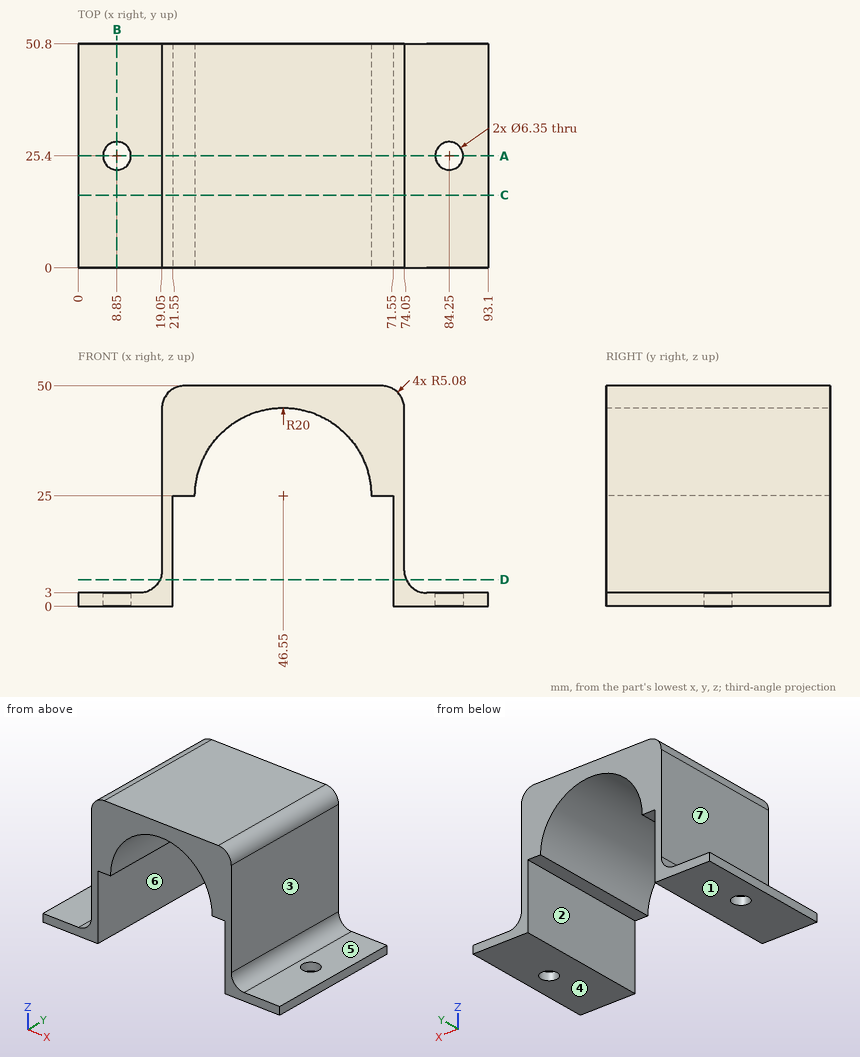
Geometry: see drawing. Coordinates: mm, zero at the bounding-box minimum. A direction names the side the tool comes from. Give positions to 0.01 mm unless a question says otherwise; leave off trailing zeros. Order: outer loops, then holes, each group sorted by start corner. A loop starts at its lowest first (then second) coordinate and runs counter-clockwise, first axis right, second up.
1. Pin query (flat end, axial travel): pin 1 Ø10 at (x, y) = (38.5, 27.5) entering from -Z; pin 2 Ø11 at (y, z) = (19.5, 21) entering from +X; pin 3 Ø8 at (x, y) = (76.5, 18) entering from +Z. Return the tip coordinate at first contact, or that it passes through.
Computed:
pin 1: stops at z = 40.16
pin 2: stops at x = 74.05
pin 3: stops at z = 48.57
2. Draft query along X for the marked faces 1, 2 and 3. Return one class per face: released by +X, released by -X, zero draft, split by the parting line, or undercut.
Computed:
face 1: zero draft
face 2: undercut
face 3: released by +X
3. Line query: probe 1 along Y at (x, z) = (84, 1); probe 2 along X at (y, z) = (15.5, 11); probe 3 along Z at (x, y) = (87, 11.5). Output: solid intervals per line, ascending.
Computed:
probe 1: y = 0 to 22.23, 28.57 to 50.8
probe 2: x = 19.05 to 21.55, 71.55 to 74.05
probe 3: z = 0 to 3
4. Cut plane A-A (y = 25.4). Return loops of the section in (x, z) (3 decimals).
Computed:
outline: (0, 0) - (5.675, 0) - (5.675, 3) - (0, 3) - close; (12.025, 0) - (21.55, 0) - (21.55, 25) - (26.55, 25) arc R20 cw to (66.55, 25) - (71.55, 25) - (71.55, 0) - (81.075, 0) - (81.075, 3) - (79.13, 3) arc R5.08 cw to (74.05, 8.08) - (74.05, 44.92) arc R5.08 ccw to (68.97, 50) - (24.13, 50) arc R5.08 ccw to (19.05, 44.92) - (19.05, 8.08) arc R5.08 cw to (13.97, 3) - (12.025, 3) - close; (87.425, 0) - (93.1, 0) - (93.1, 3) - (87.425, 3) - close
5. Cut plane C-C (y = 16.5). Return loops of the section in (x, z).
Computed:
outline: (0, 0) - (21.55, 0) - (21.55, 25) - (26.55, 25) arc R20 cw to (66.55, 25) - (71.55, 25) - (71.55, 0) - (93.1, 0) - (93.1, 3) - (79.13, 3) arc R5.08 cw to (74.05, 8.08) - (74.05, 44.92) arc R5.08 ccw to (68.97, 50) - (24.13, 50) arc R5.08 ccw to (19.05, 44.92) - (19.05, 8.08) arc R5.08 cw to (13.97, 3) - (0, 3) - close
6. Set-up query: the marked faces 4, 5, 6 and 7. Return all of +Z, -Z, +X, -X, +Y, -Y with unobstructed straight access to the full face (end or side cutting, diameter ignored); none if empty.
Computed:
face 4: -Z, +X, -X, +Y, -Y
face 5: +Z, +X, +Y, -Y
face 6: -Z, +Y, -Y
face 7: +Z, -X, +Y, -Y
7. Cut plane D-D (z = 6). Return loops of the section in (x, y), and give its area (3 significant figures).
Computed:
outline: (18.6, 0) - (21.55, 0) - (21.55, 50.8) - (18.6, 50.8) - close; (71.55, 0) - (74.5, 0) - (74.5, 50.8) - (71.55, 50.8) - close
area: 299 mm2
8. Cut plane B-B (x = 8.85). Return loops of the section in (y, z) (3 decimals), and give its area (3 significant figures).
Computed:
outline: (0, 0) - (22.225, 0) - (22.225, 3) - (0, 3) - close; (28.575, 0) - (50.8, 0) - (50.8, 3) - (28.575, 3) - close
area: 133 mm2
